Work out the finished part from the listing and answer in its coordinate system (mm). Face numbers are marked on the shaded views. A direction names the side the tool comes from. Give positions to 0.01 mm unless a question says otherwise; leave off trailing zeros. Loops run counter-clockwise (first coordinate to the right, second up) from the corner with the lowest first, then second, coordinate; pieces in that order, holes last. Notation, with made-up numbers: (48, -3.5) - (86, -3.5) arc R22 ccw to (86, 30.5) - close; hole circle Ø6 at (11.25, 19.25). An arc over 180 degrees is marked (long way). Use one line per item in the form item = value. Start each with the question number.
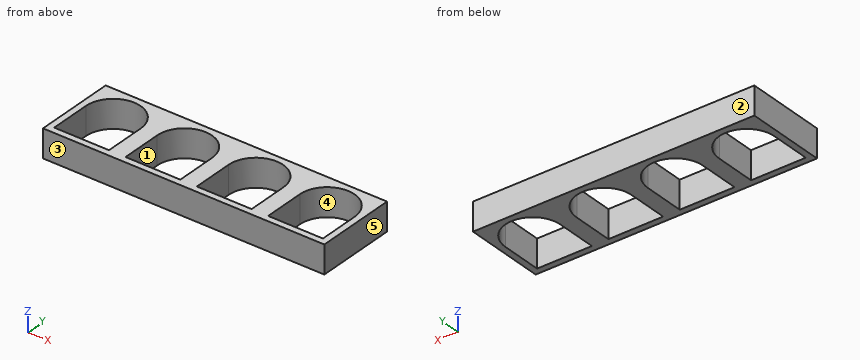
from build123d import *

# Parameters (mm, degrees)
SKETCH2_W           = 100.2
SKETCH2_H           = 28.75
BOSS_EXTRUDE1_DEPTH = 10


with BuildPart() as part:
    # Sketch2 → Boss-Extrude1 (new body)
    with BuildSketch(Plane.XY):
        with Locations((38.1, -2.375)):
            Rectangle(SKETCH2_W, SKETCH2_H)
        with BuildLine():
            Line((-9.75, -14.5), (-9.75, 0))
            ThreePointArc((-9.75, 0), (0, 9.75), (9.75, 0))
            Line((9.75, 0), (9.75, -14.5))
            Line((9.75, -14.5), (-9.75, -14.5))
        make_face(mode=Mode.SUBTRACT)
        with BuildLine():
            Line((15.65, -14.5), (15.65, 0))
            ThreePointArc((15.65, 0), (25.4, 9.75), (35.15, 0))
            Line((35.15, 0), (35.15, -14.5))
            Line((35.15, -14.5), (15.65, -14.5))
        make_face(mode=Mode.SUBTRACT)
        with BuildLine():
            Line((41.05, -14.5), (41.05, 0))
            ThreePointArc((41.05, 0), (50.8, 9.75), (60.55, 0))
            Line((60.55, 0), (60.55, -14.5))
            Line((60.55, -14.5), (41.05, -14.5))
        make_face(mode=Mode.SUBTRACT)
        with BuildLine():
            Line((66.45, -14.5), (66.45, 0))
            ThreePointArc((66.45, 0), (76.2, 9.75), (85.95, 0))
            Line((85.95, 0), (85.95, -14.5))
            Line((85.95, -14.5), (66.45, -14.5))
        make_face(mode=Mode.SUBTRACT)
    extrude(amount=BOSS_EXTRUDE1_DEPTH)


solid = part.part
1) A cutting plane is placed at D-D (x = 59). Give the vertices of the cut face in (y, z).
2) Determine the mould class of the marked faces 3, 4 and 5 for opening direction X: released by +X, released by -X, zero draft, split by the parting line, or undercut.
3) A cutting plane is placed at A-A (x = 25.4). Give the vertices of the cut face in (y, z).
4) A cutting plane is placed at C-C (z = 1.5). Give the vertices of the cut face in (x, y).
5) A tool of negligible diameter and unlimited length cuts with its end or side. For the marked faces 1 and 2, from which of +Z, -Z, +X, -X, +Y, -Y can it reach the whole face along a straight path? Write none if from no direction.
6) A cutting plane is placed at B-B (y = -10). Give the vertices of the cut face in (x, z), plus the area to 3 significant figures.
7) A flat-ended cylindrical pin translates along its axis: pin 1 Ø12 at (x, y) = (73.5, 2) entering from +Z. Find the tip coordinate at first contact, or state that the pin passes through.
8) Find the intervals of material crossed by probe 1 along X at (y, z) = (-13.5, 8.5); probe 2 along Y at (x, z) = (54, 5.75); probe 3 along X at (y, z) = (8.5, 3), in increasing order.
Answer sheet:
q1.outline = (-16.75, 0) - (-14.5, 0) - (-14.5, 10) - (-16.75, 10) - close; (5.27, 0) - (12, 0) - (12, 10) - (5.27, 10) - close
q2.face_3 = zero draft
q2.face_4 = undercut
q2.face_5 = released by +X
q3.outline = (-16.75, 0) - (-14.5, 0) - (-14.5, 10) - (-16.75, 10) - close; (9.75, 0) - (12, 0) - (12, 10) - (9.75, 10) - close
q4.outline = (-12, -16.75) - (88.2, -16.75) - (88.2, 12) - (-12, 12) - close; hole (-9.75, -14.5) - (9.75, -14.5) - (9.75, 0) arc R9.75 ccw to (-9.75, 0) - close; hole (15.65, -14.5) - (35.15, -14.5) - (35.15, 0) arc R9.75 ccw to (15.65, 0) - close; hole (41.05, -14.5) - (60.55, -14.5) - (60.55, 0) arc R9.75 ccw to (41.05, 0) - close; hole (66.45, -14.5) - (85.95, -14.5) - (85.95, 0) arc R9.75 ccw to (66.45, 0) - close
q5.face_1 = +Z, -Z
q5.face_2 = +Z, -Z, +X, -X, +Y
q6.outline = (-12, 0) - (-9.75, 0) - (-9.75, 10) - (-12, 10) - close; (9.75, 0) - (15.65, 0) - (15.65, 10) - (9.75, 10) - close; (35.15, 0) - (41.05, 0) - (41.05, 10) - (35.15, 10) - close; (60.55, 0) - (66.45, 0) - (66.45, 10) - (60.55, 10) - close; (85.95, 0) - (88.2, 0) - (88.2, 10) - (85.95, 10) - close
q6.area = 222 mm²
q7.pin_1 = through
q8.probe_1 = -12 to -9.75, 9.75 to 15.65, 35.15 to 41.05, 60.55 to 66.45, 85.95 to 88.2
q8.probe_2 = -16.75 to -14.5, 9.21 to 12
q8.probe_3 = -12 to -4.78, 4.78 to 20.62, 30.18 to 46.02, 55.58 to 71.42, 80.98 to 88.2
